Source: CAD feature listing. Evaluate the final solid. Frame: model axes, mm. A direction names the side the tool comes from. Give positions to 0.01 mm unless a question says otherwise; leave off trailing zeros. Loops run counter-clockwise (first coordinate to the right, second up) from the corner with the lowest first, then second, coordinate; pieces in that order, holes last.
```python
from build123d import *

# Parameters (mm, degrees)
SKETCH_1_W      = 15
SKETCH_1_H      = 15
EXTRUDE_1_DEPTH = 2
FILLET_1_R      = 1
SKETCH_2_W      = 1.2
SKETCH_2_H      = 3
EXTRUDE_2_DEPTH = 4
FILLET_2_R      = 0.3


with BuildPart() as part:
    # 草图1 → 凸台-拉伸1 (new body)
    with BuildSketch(Plane(origin=(0, 0, 0), x_dir=(1, 0, 0), z_dir=(0, 1, 0))):
        with Locations((30.528568239, 7.5)):
            Rectangle(SKETCH_1_W, SKETCH_1_H)
    extrude(amount=EXTRUDE_1_DEPTH)

    # 圆角1
    fillet_1_edges = [part.edges().sort_by_distance(p)[0] for p in [
        (38.028568239, 2, -7.5),
        (30.528568239, 2, -15),
        (23.028568239, 2, -7.5),
        (23.028568239, 1, -15),
        (38.028568239, 1, -15),
        (38.028568239, 1, 0),
        (23.028568239, 1, 0),
        (30.528568239, 2, 0),
    ]]
    fillet(fillet_1_edges, radius=FILLET_1_R)

    # 草图2 → 凸台-拉伸2 (add)
    with BuildSketch(Plane.XZ):
        with Locations((33.378568239, -7.5)):
            Rectangle(SKETCH_2_W, SKETCH_2_H)
        with Locations((27.678568239, -7.5)):
            Rectangle(SKETCH_2_W, SKETCH_2_H)
    extrude(amount=EXTRUDE_2_DEPTH)

    # 圆角2
    fillet_2_edges = [part.edges().sort_by_distance(p)[0] for p in [
        (30.528568239, 0, 0),
        (38.028568239, 0, -7.5),
        (23.028568239, 0, -7.5),
        (30.528568239, 0, -15),
        (23.321461458, 0, -0.292893219),
        (37.73567502, 0, -0.292893219),
        (23.321461458, 0, -14.707106781),
        (37.73567502, 0, -14.707106781),
        (28.278568239, 0, -7.5),
        (27.678568239, 0, -6),
        (27.078568239, 0, -7.5),
        (27.678568239, 0, -9),
        (28.278568239, -4, -7.5),
        (27.678568239, -4, -6),
        (27.078568239, -4, -7.5),
        (27.678568239, -4, -9),
        (33.978568239, 0, -7.5),
        (33.378568239, 0, -6),
        (32.778568239, 0, -7.5),
        (33.378568239, 0, -9),
        (33.978568239, -4, -7.5),
        (33.378568239, -4, -6),
        (32.778568239, -4, -7.5),
        (33.378568239, -4, -9),
    ]]
    fillet(fillet_2_edges, radius=FILLET_2_R)


solid = part.part
```
(1) Mould query, pull axis X, two halves, no side actions, for faces 1 (the flat face through (32.779, -2, -8)), 2 (the flat face through (33.979, -2, -8)), 3 (the cylindrical face through (30.62, 1.699, -14.715)). Classes: pulls with the +X half, pulls with the -X half, needs draft (parallel to the pull), parting line crosses it, or undercut.
A:
face 1: undercut
face 2: pulls with the +X half
face 3: needs draft
(2) Ray query, line 1 along Y through (x, z) = (36, -10); line 2 along X through (y, z) = (1.4, -6.25); line 3 along Y through (x, z) = (33, -7.75). Return the intervals inside material, ascending.
A:
line 1: y = 0 to 2
line 2: x = 23.11 to 37.95
line 3: y = -3.99 to 2
(3) Section C-C, the plane x = 33.5. Return the cut outline in (y, z).
A:
outline: (-4, -8.7) arc R0.3 ccw to (-3.7, -9) - (-0.3, -9) arc R0.3 cw to (0, -9.3) - (0, -14.7) arc R0.3 ccw to (0.3, -15) - (1, -15) arc R1 ccw to (2, -14) - (2, -1) arc R1 ccw to (1, 0) - (0.3, 0) arc R0.3 ccw to (0, -0.3) - (0, -5.7) arc R0.3 cw to (-0.3, -6) - (-3.7, -6) arc R0.3 ccw to (-4, -6.3) - close
(4) Reachability of faces 4 (the flat face through (27.079, -2, -8)), 5 (the flat face through (28.279, -2, -8)), 6 (the flat face through (28, -2, -9)), 7 (the cylindrical face through (37.74, 1.7, -7.59)), 8 (the flat face through (33, -2, -6)) from +Z, -Z, +X, -X, +Y, -Y: full face, straight path, thin tool, end or side. Return the list, or none.
A:
face 4: +Z, -Z, -X, -Y
face 5: +Z, -Z, -Y
face 6: -Z, +X, -X, -Y
face 7: +Z, -Z, +X, +Y
face 8: +Z, +X, -X, -Y
(5) Section B-B, the plane z = -4.5. Return the cut outline in (x, y).
A:
outline: (23.03, 0.3) arc R0.3 ccw to (23.33, 0) - (37.73, 0) arc R0.3 ccw to (38.03, 0.3) - (38.03, 1) arc R1 ccw to (37.03, 2) - (24.03, 2) arc R1 ccw to (23.03, 1) - close
(6) Section D-D, the plane y = 1.5. Return the cut outline in (x, z).
A:
outline: (23.16, -14) arc R0.87 ccw to (24.03, -14.87) - (37.03, -14.87) arc R0.87 ccw to (37.89, -14) - (37.89, -1) arc R0.87 ccw to (37.03, -0.13) - (24.03, -0.13) arc R0.87 ccw to (23.16, -1) - close
(7) First-contact query: pin 1 (1.3 mm diameter, centred on x = 33.5, y = -3, fed in from -Z); pin 2 (3 mm diameter, centred on x = 30, z = -4, fed in from -Y); pin 3 (1.5 mm diameter, centred on y = -2, z = -7.5, fed in from -X). Flat tips, straight axial feed; report the tip coordinate or a pass-through.
A:
pin 1: stops at z = -9
pin 2: stops at y = 0
pin 3: stops at x = 27.08
(8) Section A-A, the plane y = -2.3. Return the cut outline in (x, z), then the cut area to 3 significant figures.
A:
outline: (27.08, -9) - (28.28, -9) - (28.28, -6) - (27.08, -6) - close; (32.78, -9) - (33.98, -9) - (33.98, -6) - (32.78, -6) - close
area: 7.20 mm2
